CAD build for the part. Positions are in the model's coordinates, mm. A direction names the side the tool comes from. Give positions to 0.01 mm unless a question says otherwise; leave off trailing zeros. Write each loop counter-clockwise with the first axis right and the second up, starting at its lowest first coordinate (ties: lowest second). Pieces come first, ordered by that corner, then holes. Notation, with made-up numbers: (8.5, 55) - (44.5, 55) arc R17 cw to (44.5, 76) - close; hole circle Ø5 at (-21, 41.25). An arc over 180 degrees is marked (long way). Put each result on its own line as item: value. Start each with the question number.
1. Cut at D-D on y = -16.5. List the corners of the cut face in (x, z), and give its area (3 significant figures).
2. Mould opens along X. For faces 1 (the flat face through (-6.15, -8.29, 4.93)), 2 (the flat face through (-21.55, 12.675, 4.93)), 3 (the flat face through (21.55, -12.675, 4.93)) say: +X half, -X half, draft (parallel to the pull), parting line (faces both ways), or undercut.
3. Cut at C-C on x = -4. List the corners of the cut face in (y, z), and give its area (3 significant figures).
4. Wall check: line 1 (Y direction, x = -5.5, z = 7); line 2 (X direction, y = -4.5, z = 2.5); line 3 (Y direction, x = -4.5, z = 1.25). Give the ranges that are in metal, low to high.
5. Cut at A-A on y = 1. List the corners of the cut face in (x, z).
6. Drop flat-ended pins along their axis: pin 1 (3 mm diameter, centred on y = -15.5, z = 5.5, fed in from +X); pin 2 (6 mm diameter, centred on y = 3.5, z = 4, fed in from -X); pin 3 (4 mm diameter, centred on x = 18, z = 3.5, fed in from -Y). Give the stop position or say it passes through.
7. Tool access for faces 4 (the flat face through (21.752, 12.325, 4.93)), 5 (the flat face through (6, -8.4, 4.9)): list every direction of +Z, -Z, +X, -X, +Y, -Y with a clear straight run to the whole face (end or side of a thin tool).
8. Cut at B-B on z = 1. List the corners of the cut face in (x, y).
from build123d import *

# Parameters (mm, degrees)
EXTRUDE_DEPTH = 10


with BuildPart() as part:
    # Sketch → Extrude (new body)
    with BuildSketch(Plane.XY):
        Polygon((28.867513, 0), (14.433757, 25), (-14.433757, 25), (-28.867513, 0), (-14.433757, -25), (14.433757, -25), align=None)
        Polygon((7.5, 10.322864), (-7.5, 10.322864), (-12.135255, -3.942983), (0, -12.759762), (12.135255, -3.942983), align=None, mode=Mode.SUBTRACT)
    extrude(amount=EXTRUDE_DEPTH)


solid = part.part
Report:
1. outline: (-19.34, 0) - (19.34, 0) - (19.34, 10) - (-19.34, 10) - close
1. area: 387 mm²
2. face 1: undercut
2. face 2: -X half
2. face 3: +X half
3. outline: (-25, 0) - (-9.85, 0) - (-9.85, 10) - (-25, 10) - close; (10.32, 0) - (25, 0) - (25, 10) - (10.32, 10) - close
3. area: 298 mm²
4. line 1: y = -25 to -8.76, 10.32 to 25
4. line 2: x = -26.27 to -11.37, 11.37 to 26.27
4. line 3: y = -25 to -9.49, 10.32 to 25
5. outline: (-28.29, 0) - (-10.53, 0) - (-10.53, 10) - (-28.29, 10) - close; (10.53, 0) - (28.29, 0) - (28.29, 10) - (10.53, 10) - close
6. pin 1: stops at x = 20.78
6. pin 2: stops at x = -28.58
6. pin 3: stops at y = -22.29
7. face 4: +Z, -Z, +X, +Y
7. face 5: +Z, -Z
8. outline: (-28.87, 0) - (-14.43, -25) - (14.43, -25) - (28.87, 0) - (14.43, 25) - (-14.43, 25) - close; hole (-12.14, -3.94) - (0, -12.76) - (12.14, -3.94) - (7.5, 10.32) - (-7.5, 10.32) - close
